Autodesk Inventor part; units mm, degrees
ref_plane "YZ Plane" through (0, 0, 0) normal (1, 0, 0) x (0, 1, 0)
ref_plane "XZ Plane" through (0, 0, 0) normal (0, 1, 0) x (-1, 0, 0)
ref_plane "XY Plane" through (0, 0, 0) normal (0, 0, 1) x (1, 0, 0)
sketch "Sketch1" plane through (0, 0, 0) normal (0, 0, 1) x (1, 0, 0)
  line L0 (-16, -12.5) -> (16, -12.5)
  line L1 (16, -12.5) -> (16, 12.5)
  line L2 (16, 12.5) -> (13, 12.5)
  line L3 (13, 12.5) -> (13, -9.5)
  line L4 (13, -9.5) -> (-13, -9.5)
  line L5 (-13, -9.5) -> (-13, 12.5)
  line L6 (-13, 12.5) -> (-16, 12.5)
  line L7 (-16, 12.5) -> (-16, -12.5)
  point P0 (0, 0)
  dimension "d0" = 32
  dimension "d1" = 25
  dimension "d2" = 3
  dimension "d3" = 90
  dimension "d4" = 22
  dimension "d5" = 26
  dimension "d6" = 22
  dimension "d7" = 3
  dimension "d8" = 25
  dimension "d10" = 12.5
  dimension "d11" = 16
extrude "Extrusion1" add sketch "Sketch1" against normal blind 609.6
chamfer "Chamfer1" distance 25 angle 30 1 edges at (14.5, 12.5, 0) measured on face at (4.3333, -11.5, 0)
chamfer "Chamfer2" distance 25 angle 30 1 edges at (14.5, 12.5, -609.6) measured on face at (4.3333, -11.5, -609.6)
equation "\"d5\" = d0 - 2 * d2"
properties part number "Chassis Edge"
For this review, take the finished solid that the model builds, in its own axes (mm). A direction names the side the tool comes from. Give positions to 0.01 mm unless a question says otherwise; leave off trailing zeros. Loops run counter-clockwise (first coordinate to the right, second up) from the corner with the lowest first, then second, coordinate; pieces in that order, holes last.
Item 1: Insertion check: pin 1 (12 mm diameter, centred on x = 4.5, z = -398.5, fed in from +Y). The pin has a flat end and moves straight along its axis. Give the tip position at first contact, or say it passes through.
Item 2: Tool access review of faces 5 (the flat face through (-16, 0, -301)), 6 (the flat face through (13, 2, -301)): name each direction out of +Z, -Z, +X, -X, +Y, -Y from which nothing blocks a thin tool from reaching the whole face with its end or side.
Item 3: For line 1 along X through (y, z) = (-5, -561.5); line 2 along Y through (x, z) = (-12.5, -33), list the stretches that pass through material, from the lowest coordinate up.
Item 4: Take a section at A-A, the plane y = -5.25. State the section outline as (x, z) points.
Item 5: Draft analysis for pull direction X (two halves, no side actions). For faces 1 (the flat face through (16, 0, -301)), 2 (the flat face through (-13, 1, -301)), 3 (the flat face through (0, -9.5, -301)), 4 (the flat face through (-1.26, -10.13, -1.37)), state which applies: +X half, -X half, draft (parallel to the pull), parting line (faces both ways), or undercut.
Item 6: Take a section at B-B, the plane z = -135. State the section outline as (x, y) points.
Calculated:
1. pin 1: stops at y = -9.5
2. face 5: +Z, -Z, -X, +Y, -Y
2. face 6: +Z, -Z, +Y
3. line 1: x = -16 to -13, 13 to 16
3. line 2: y = -12.5 to -9.5
4. outline: (-16, -605.41) - (-13, -605.41) - (-13, -4.19) - (-16, -4.19) - close; (13, -605.41) - (16, -605.41) - (16, -4.19) - (13, -4.19) - close
5. face 1: +X half
5. face 2: undercut
5. face 3: undercut
5. face 4: draft
6. outline: (-16, -12.5) - (16, -12.5) - (16, 12.5) - (13, 12.5) - (13, -9.5) - (-13, -9.5) - (-13, 12.5) - (-16, 12.5) - close
